```python
from build123d import *
from OCP.BRepFilletAPI import BRepFilletAPI_MakeChamfer

# Parameters (mm, degrees)
SM_BASE_FLANGE_1_DEPTH = 130
SKETCH_6_R             = 2.1
CUT_EXTRUDE_1_DEPTH    = 147.989795564
PATTERN_LINEAR_1_COUNT = 2
PATTERN_LINEAR_1_PITCH = 45
CHAMFER_1_SIZE         = 10
CHAMFER_1_SIZE2        = 40
CHAMFER_2_SIZE         = 40
CHAMFER_2_SIZE2        = 10
FILLET_1_R             = 5
SKETCH_9_W             = 53.5268
SKETCH_9_H             = 2
EXTRUDE_1_DEPTH        = 15
CHAMFER_5_SIZE         = 10
CHAMFER_5_SIZE_2       = 15
SKETCH_11_W            = 53.5268
SKETCH_11_H            = 2
EXTRUDE_2_DEPTH        = 25
CHAMFER_6_SIZE         = 15


# Read off the part's stored shape, not the designer's step: 基材-凸緣1
with BuildPart() as part:
    # 基材-凸緣1 outline → 基材-凸緣1 (new body)
    with BuildSketch(Plane.XY):
        with BuildLine():
            Line((29.5, 0.7366), (29.5, 35))
            Line((29.5, 35), (27.5, 35))
            Line((27.5, 35), (27.5, 0.7366))
            ThreePointArc((27.5, 0.7366), (27.284254855, 0.215745145), (26.7634, 0))
            Line((26.7634, 0), (-26.7634, 0))
            ThreePointArc((-26.7634, 0), (-27.284254855, 0.215745145), (-27.5, 0.7366))
            Line((-27.5, 0.7366), (-27.5, 35))
            Line((-27.5, 35), (-29.5, 35))
            Line((-29.5, 35), (-29.5, 0.7366))
            ThreePointArc((-29.5, 0.7366), (-28.698468417, -1.198468417), (-26.7634, -2))
            Line((-26.7634, -2), (26.7634, -2))
            ThreePointArc((26.7634, -2), (28.698468417, -1.198468417), (29.5, 0.7366))
        make_face()
    extrude(amount=SM_BASE_FLANGE_1_DEPTH)

    # 草圖6 → 除料-伸長1 (cut, through all)
    with BuildSketch(Plane.ZY.offset(29.5)):
        with Locations((72, 10)):
            Circle(SKETCH_6_R)
    cut_extrude_1 = extrude(amount=-CUT_EXTRUDE_1_DEPTH, mode=Mode.SUBTRACT)

    # 直線複製排列1: 除料-伸長1 ×2
    with Locations(*[(0, 0, -i * PATTERN_LINEAR_1_PITCH) for i in range(1, PATTERN_LINEAR_1_COUNT)]):
        add(cut_extrude_1, mode=Mode.SUBTRACT)

    # 導角1
    chamfer_1_edges = [part.edges().sort_by_distance(p)[0] for p in [
        (-28.5, 35, 130),
        (28.5, 35, 130),
    ]]
    chamfer_1_side = [part.faces().sort_by_distance(p)[0] for p in [
        (0, -1.303580586, 130),
    ]]
    chamfer(chamfer_1_edges, length=CHAMFER_1_SIZE, length2=CHAMFER_1_SIZE2, reference=chamfer_1_side[0])

    # 導角2: one chamfer whose edges measure the first distance from different faces: ONE call of the kernel's chamfer builder (chamfer() names one face for all edges)
    chamfer_2_edges_1 = [part.edges().sort_by_distance(p)[0] for p in [
        (-28.5, 35, 0),
    ]]
    chamfer_2_side_1 = [part.faces().sort_by_distance(p)[0] for p in [
        (-28.5, 35, 45),
    ]]
    chamfer_2_edges_2 = [part.edges().sort_by_distance(p)[0] for p in [
        (28.5, 35, 0),
    ]]
    chamfer_2_side_2 = [part.faces().sort_by_distance(p)[0] for p in [
        (28.5, 35, 45),
    ]]
    chamfer_2 = BRepFilletAPI_MakeChamfer(part.part.solid().wrapped)
    for e in chamfer_2_edges_1:
        chamfer_2.Add(CHAMFER_2_SIZE, CHAMFER_2_SIZE2, e.wrapped, chamfer_2_side_1[0].wrapped)  # the first distance lies on this face
    for e in chamfer_2_edges_2:
        chamfer_2.Add(CHAMFER_2_SIZE, CHAMFER_2_SIZE2, e.wrapped, chamfer_2_side_2[0].wrapped)  # the first distance lies on this face
    add(Compound.cast(chamfer_2.Shape()), mode=Mode.REPLACE)

    # 圓角1
    fillet_1_edges = [part.edges().sort_by_distance(p)[0] for p in [
        (28.5, 35, 90),
        (28.5, 25, 130),
        (-28.5, 35, 90),
        (-28.5, 25, 130),
        (-28.5, 25, 0),
        (-28.5, 35, 40),
        (28.5, 25, 0),
        (28.5, 35, 40),
    ]]
    fillet(fillet_1_edges, radius=FILLET_1_R)

    # 草圖9 → 填料-伸長1 (add)
    with BuildSketch(Plane.XY.offset(130)):
        with Locations((0, -1)):
            Rectangle(SKETCH_9_W, SKETCH_9_H)
    extrude(amount=EXTRUDE_1_DEPTH)

    # 導角5
    chamfer_5_edges_1 = [part.edges().sort_by_distance(p)[0] for p in [
        (-26.7634, -1, 145),
    ]]
    chamfer_5_side_1 = [part.faces().sort_by_distance(p)[0] for p in [
        (-26.5634, -1, 145),
    ]]
    chamfer_5_edges_2 = [part.edges().sort_by_distance(p)[0] for p in [
        (26.7634, -1, 145),
    ]]
    chamfer_5_side_2 = [part.faces().sort_by_distance(p)[0] for p in [
        (26.7634, -1, 144.8),
    ]]
    chamfer_5 = BRepFilletAPI_MakeChamfer(part.part.solid().wrapped)
    for e in chamfer_5_edges_1:
        chamfer_5.Add(CHAMFER_5_SIZE - 0.0001, CHAMFER_5_SIZE_2 - 0.0001, e.wrapped, chamfer_5_side_1[0].wrapped)
    for e in chamfer_5_edges_2:
        chamfer_5.Add(CHAMFER_5_SIZE_2 - 0.0001, CHAMFER_5_SIZE - 0.0001, e.wrapped, chamfer_5_side_2[0].wrapped)
    add(Compound.cast(chamfer_5.Shape()), mode=Mode.REPLACE)  # a hair under: the kernel refuses the full size

    # 草圖11 → 填料-伸長2 (add)
    with BuildSketch(Plane(origin=(0, 0, 0), x_dir=(-1, 0, 0), z_dir=(0, 0, -1))):
        with Locations((0, -1)):
            Rectangle(SKETCH_11_W, SKETCH_11_H)
    extrude(amount=EXTRUDE_2_DEPTH)

    # 導角6
    chamfer_6_edges = [part.edges().sort_by_distance(p)[0] for p in [
        (26.7634, -1, -25),
        (-26.7634, -1, -25),
    ]]
    chamfer(chamfer_6_edges, length=CHAMFER_6_SIZE)


solid = part.part
```
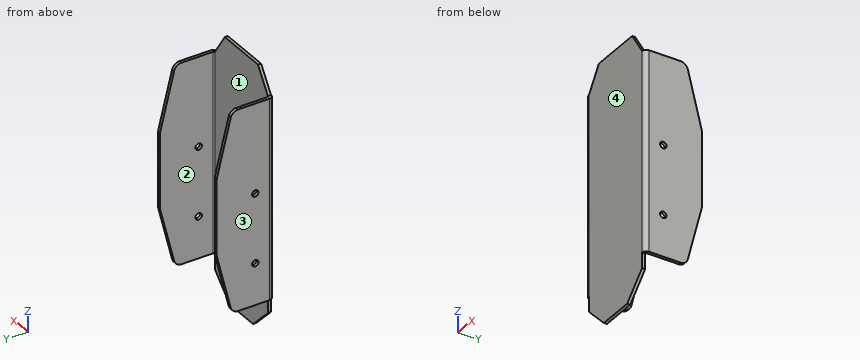
Read the model definition and answer for the solid it produces. Units are mm, in the model's axes. Face numbers are marked on the shaded views. Round coordinates to 2 decimals unless told otherwise and drop trailing zeros. Write each loop counter-clockwise with the first axis right and the second up, starting at its lowest first coordinate (ties: lowest second). Pieces come first, ordered by that corner, then holes. Notation, with made-up numbers: (66.5, 62) -> (75.5, 62) arc R23 cw to (75.5, 86) -> close; hole circle Ø1 at (-11, -31.5). An arc over 180 degrees is marked (long way). Answer in a Markdown table with one row per item. Add a question column.
1) Find section A-A, the plane y = 10. Determine the outline of the cut face in (x, z).
2) Find section B-B, the plane z = 72. Determine the outline of the cut face in (x, y).
3) Find section D-D, the plane z = 116. Determine the outline of the cut face in (x, y).
4) Find section C-C, the plane z = 27. Determine the outline of the cut face in (x, y).
5) Determine the mould class of the marked faces 1, 2, 3 and 4 for opening direction X: pulls with the +X half, pulls with the -X half, needs draft (parallel to the pull), parting line crosses it, or undercut.
6) Given P1, Ø1, axis at y = -1, z = -4.5, coming from the -X side; P2, Ø0.6, axis at y = -0.5, z = -4, coming from the +X side; P3, Ø1.5, axis at x = 19, z = 61, coming from the +Y side, each flat-ended and moving along its own axis, determine where each tip first touches the part or whether it passes through.
7) Consider line 1 (X direction, y = 26.5, z = 21); line 2 (Y direction, x = -7, z = 10); line 3 (Y direction, x = 28.3, z = 72). Determine where each line is inside the solid, lowest interval first.
Findings below:
| question | item | result |
|---|---|---|
| 1 | outline | (-29.5, 0) -> (-27.5, 0) -> (-27.5, 24.9) -> (-29.5, 24.9) -> close; (-29.5, 29.1) -> (-27.5, 29.1) -> (-27.5, 69.9) -> (-29.5, 69.9) -> close; (-29.5, 74.1) -> (-27.5, 74.1) -> (-27.5, 130) -> (-29.5, 130) -> close; (27.5, 0) -> (29.5, 0) -> (29.5, 24.9) -> (27.5, 24.9) -> close; (27.5, 29.1) -> (29.5, 29.1) -> (29.5, 69.9) -> (27.5, 69.9) -> close; (27.5, 74.1) -> (29.5, 74.1) -> (29.5, 130) -> (27.5, 130) -> close |
| 2 | outline | (-29.5, 0.74) arc R2.74 ccw to (-26.76, -2) -> (26.76, -2) arc R2.74 ccw to (29.5, 0.74) -> (29.5, 7.9) -> (27.5, 7.9) -> (27.5, 0.74) arc R0.74 cw to (26.76, 0) -> (-26.76, 0) arc R0.74 cw to (-27.5, 0.74) -> (-27.5, 7.9) -> (-29.5, 7.9) -> close; (-29.5, 12.1) -> (-27.5, 12.1) -> (-27.5, 35) -> (-29.5, 35) -> close; (27.5, 12.1) -> (29.5, 12.1) -> (29.5, 35) -> (27.5, 35) -> close |
| 3 | outline | (-29.5, 0.74) arc R2.74 ccw to (-26.76, -2) -> (26.76, -2) arc R2.74 ccw to (29.5, 0.74) -> (29.5, 28.5) -> (27.5, 28.5) -> (27.5, 0.74) arc R0.74 cw to (26.76, 0) -> (-26.76, 0) arc R0.74 cw to (-27.5, 0.74) -> (-27.5, 28.5) -> (-29.5, 28.5) -> close |
| 4 | outline | (-29.5, 0.74) arc R2.74 ccw to (-26.76, -2) -> (26.76, -2) arc R2.74 ccw to (29.5, 0.74) -> (29.5, 7.9) -> (27.5, 7.9) -> (27.5, 0.74) arc R0.74 cw to (26.76, 0) -> (-26.76, 0) arc R0.74 cw to (-27.5, 0.74) -> (-27.5, 7.9) -> (-29.5, 7.9) -> close; (-29.5, 12.1) -> (-27.5, 12.1) -> (-27.5, 31.75) -> (-29.5, 31.75) -> close; (27.5, 12.1) -> (29.5, 12.1) -> (29.5, 31.75) -> (27.5, 31.75) -> close |
| 5 | face 1 | undercut |
| 5 | face 2 | undercut |
| 5 | face 3 | pulls with the -X half |
| 5 | face 4 | needs draft |
| 6 | P1 | x = -26.76 |
| 6 | P2 | x = 26.76 |
| 6 | P3 | y = 0 |
| 7 | line 1 | -29.5 to -27.5, 27.5 to 29.5 |
| 7 | line 2 | -2 to 0 |
| 7 | line 3 | -1.53 to 7.9, 12.1 to 35 |
